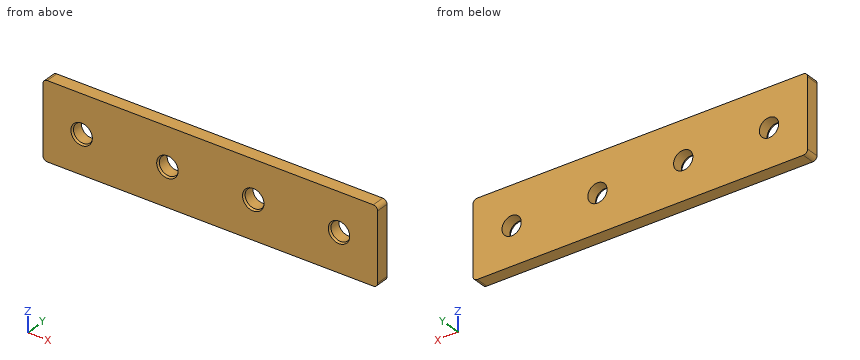
from build123d import *

# Parameters (mm, degrees)
F0_R     = 4.5
F1_DEPTH = 6
F2_SIZE2 = 0.5
F2_SIZE  = 1


with BuildPart() as f1:
    # F0 (on Front) → F1 (new body)
    with BuildSketch(Plane.XZ):
        with BuildLine():
            Line((136, 18), (-16, 18))
            ThreePointArc((-16, 18), (-17.414214, 17.414214), (-18, 16))
            Line((-18, 16), (-18, -16))
            ThreePointArc((-18, -16), (-17.414214, -17.414214), (-16, -18))
            Line((-16, -18), (136, -18))
            ThreePointArc((136, -18), (137.414214, -17.414214), (138, -16))
            Line((138, -16), (138, 16))
            ThreePointArc((138, 16), (137.414214, 17.414214), (136, 18))
        make_face()
        Circle(F0_R, mode=Mode.SUBTRACT)
        with Locations((40, 0)):
            Circle(F0_R, mode=Mode.SUBTRACT)
        with Locations((80, 0)):
            Circle(F0_R, mode=Mode.SUBTRACT)
        with Locations((120, 0)):
            Circle(F0_R, mode=Mode.SUBTRACT)
    extrude(amount=F1_DEPTH)

    # F2
    f2_edges = [f1.edges().sort_by_distance(p)[0] for p in [
        (-4.5, -6, 0),
        (35.5, -6, 0),
        (75.5, -6, 0),
        (115.5, -6, 0),
    ]]
    chamfer(f2_edges, length=F2_SIZE, length2=F2_SIZE2)


solid = f1.part
Read the model definition and answer for the solid it produces. Units are mm, in the model's axes. Coordinates: 2 decimals unless noted, no trailing zeros. Order: outer loops, then holes, each group sorted by start corner. A loop starts at its lowest first (then second) coordinate and runs counter-clockwise, first axis right, second up. Notation, with made-up numbers: M 19.5,-10 L 37.5,-10 A25 cw 37.5,6 Z; hole C 2,-36 d11. An arc over 180 degrees is marked long. Put each result on its own line as item: value. Start each with the question number.
Item 1: Given pin 1 Ø11.5 at (x, z) = (40, 0) entering from -Y, flat-ended and moving along its own axis, determine where the tip first touches the part or whether it passes through.
Item 2: Section B-B, the plane x = 40 is taken. Determine the outline of the cut face in (y, z).
Item 3: Consider probe 1 along X at (y, z) = (-2.7, -0.5); probe 2 along Z at (x, y) = (120, -1.6); probe 3 along X at (y, z) = (-2.25, 3.5). Determine where each line is inside the solid, lowest interval first. Write a range as [from, to].
Item 4: Section C-C, the plane y = -2 is taken. Determine the outline of the cut face in (x, z).
Item 5: Section A-A, the plane z = 0 is taken. Determine the outline of the cut face in (x, y).
Computed:
1. pin 1: stops at y = -6
2. outline: M -6,-18 L 0,-18 L 0,-4.5 L -5,-4.5 L -6,-5 Z; M -6,5 L -5,4.5 L 0,4.5 L 0,18 L -6,18 Z
3. probe 1: x = [-18, -4.47], [4.47, 35.53], [44.47, 75.53], [84.47, 115.53], [124.47, 138]
3. probe 2: z = [-18, -4.5], [4.5, 18]
3. probe 3: x = [-18, -2.83], [2.83, 37.17], [42.83, 77.17], [82.83, 117.17], [122.83, 138]
4. outline: M -18,-16 A2 ccw -16,-18 L 136,-18 A2 ccw 138,-16 L 138,16 A2 ccw 136,18 L -16,18 A2 ccw -18,16 Z; hole C 0,0 d9; hole C 40,0 d9; hole C 80,0 d9; hole C 120,0 d9
5. outline: M -18,-6 L -5,-6 L -4.5,-5 L -4.5,0 L -18,0 Z; M 4.5,-5 L 5,-6 L 35,-6 L 35.5,-5 L 35.5,0 L 4.5,0 Z; M 44.5,-5 L 45,-6 L 75,-6 L 75.5,-5 L 75.5,0 L 44.5,0 Z; M 84.5,-5 L 85,-6 L 115,-6 L 115.5,-5 L 115.5,0 L 84.5,0 Z; M 124.5,-5 L 125,-6 L 138,-6 L 138,0 L 124.5,0 Z
